```python
from build123d import *

# Parameters (mm, degrees)
SKETCH1_R           = 2.6
SKETCH1_R_2         = 7.6
BOSS_EXTRUDE1_DEPTH = 1.8
FILLET1_R           = 3
FILLET2_R           = 1.4
SCALE1_SCALE        = 1.15


with BuildPart() as part:
    # Sketch1 → Boss-Extrude1 (new body)
    with BuildSketch(Plane(origin=(0, 0, 0), x_dir=(1, 0, 0), z_dir=(0, 1, 0))):
        Polygon((20.3, 35.160631394), (-20.3, 35.160631394), (-40.6, 0), (-20.3, -35.160631394), (20.3, -35.160631394), (40.6, 0), align=None)
        with Locations((-18.636201283, -32.21652123)):
            Circle(SKETCH1_R, mode=Mode.SUBTRACT)
        with Locations((18.582225165, -32.247684356)):
            Circle(SKETCH1_R, mode=Mode.SUBTRACT)
        with Locations((37.218426448, -0.031163126)):
            Circle(SKETCH1_R, mode=Mode.SUBTRACT)
        with Locations((-37.218426448, 0.031163126)):
            Circle(SKETCH1_R, mode=Mode.SUBTRACT)
        with BuildLine():
            Line((-32.142053523, 3.218057696), (-18.857946477, 26.226806032))
            Line((-18.857946477, 26.226806032), (-10.521325069, 11.78735419))
            ThreePointArc((-10.521325069, 11.78735419), (-13.68320138, 7.9), (-15.468810706, 3.218057696))
            Line((-15.468810706, 3.218057696), (-32.142053523, 3.218057696))
        make_face(mode=Mode.SUBTRACT)
        with BuildLine():
            Line((-18.857946477, -26.226806032), (-32.142053523, -3.218057696))
            Line((-32.142053523, -3.218057696), (-15.468810706, -3.218057696))
            ThreePointArc((-15.468810706, -3.218057696), (-13.68320138, -7.9), (-10.521325069, -11.78735419))
            Line((-10.521325069, -11.78735419), (-18.857946477, -26.226806032))
        make_face(mode=Mode.SUBTRACT)
        with BuildLine():
            Line((13.284107046, -29.444863729), (-13.284107046, -29.444863729))
            Line((-13.284107046, -29.444863729), (-4.947485637, -15.005411886))
            ThreePointArc((-4.947485637, -15.005411886), (0, -15.8), (4.947485637, -15.005411886))
            Line((4.947485637, -15.005411886), (13.284107046, -29.444863729))
        make_face(mode=Mode.SUBTRACT)
        with BuildLine():
            Line((32.142053523, -3.218057696), (18.857946477, -26.226806032))
            Line((18.857946477, -26.226806032), (10.521325069, -11.78735419))
            ThreePointArc((10.521325069, -11.78735419), (13.68320138, -7.9), (15.468810706, -3.218057696))
            Line((15.468810706, -3.218057696), (32.142053523, -3.218057696))
        make_face(mode=Mode.SUBTRACT)
        with BuildLine():
            Line((18.857946477, 26.226806032), (32.142053523, 3.218057696))
            Line((32.142053523, 3.218057696), (15.468810706, 3.218057696))
            ThreePointArc((15.468810706, 3.218057696), (13.68320138, 7.9), (10.521325069, 11.78735419))
            Line((10.521325069, 11.78735419), (18.857946477, 26.226806032))
        make_face(mode=Mode.SUBTRACT)
        with BuildLine():
            Line((-13.284107046, 29.444863729), (13.284107046, 29.444863729))
            Line((13.284107046, 29.444863729), (4.947485637, 15.005411886))
            ThreePointArc((4.947485637, 15.005411886), (0, 15.8), (-4.947485637, 15.005411886))
            Line((-4.947485637, 15.005411886), (-13.284107046, 29.444863729))
        make_face(mode=Mode.SUBTRACT)
        with Locations((-18.582225165, 32.247684356)):
            Circle(SKETCH1_R, mode=Mode.SUBTRACT)
        with Locations((18.636201283, 32.21652123)):
            Circle(SKETCH1_R, mode=Mode.SUBTRACT)
        with Locations((0.052857117, 0)):
            Circle(SKETCH1_R_2, mode=Mode.SUBTRACT)
    extrude(amount=BOSS_EXTRUDE1_DEPTH)

    # Fillet1
    fillet1_edges = [part.edges().sort_by_distance(p)[0] for p in [
        (40.6, 0.9, 0),
        (20.3, 0.9, 35.160631394),
        (-20.3, 0.9, 35.160631394),
        (-40.6, 0.9, 0),
        (-20.3, 0.9, -35.160631394),
        (20.3, 0.9, -35.160631394),
    ]]
    fillet(fillet1_edges, radius=FILLET1_R)

    # Fillet2
    fillet2_edges = [part.edges().sort_by_distance(p)[0] for p in [
        (-32.142053523, 0.9, -3.218057696),
        (-15.468810706, 0.9, -3.218057696),
        (-10.521325069, 0.9, -11.78735419),
        (-18.857946477, 0.9, -26.226806032),
        (-18.857946477, 0.9, 26.226806032),
        (-10.521325069, 0.9, 11.78735419),
        (-15.468810706, 0.9, 3.218057696),
        (-32.142053523, 0.9, 3.218057696),
        (13.284107046, 0.9, 29.444863729),
        (4.947485637, 0.9, 15.005411886),
        (-4.947485637, 0.9, 15.005411886),
        (-13.284107046, 0.9, 29.444863729),
        (32.142053523, 0.9, 3.218057696),
        (15.468810706, 0.9, 3.218057696),
        (10.521325069, 0.9, 11.78735419),
        (18.857946477, 0.9, 26.226806032),
        (18.857946477, 0.9, -26.226806032),
        (10.521325069, 0.9, -11.78735419),
        (15.468810706, 0.9, -3.218057696),
        (32.142053523, 0.9, -3.218057696),
        (-13.284107046, 0.9, -29.444863729),
        (-4.947485637, 0.9, -15.005411886),
        (4.947485637, 0.9, -15.005411886),
        (13.284107046, 0.9, -29.444863729),
    ]]
    fillet(fillet2_edges, radius=FILLET2_R)


with BuildPart() as part_1:
    # Scale1: scaled about (-0.003928135, 0.9, 0)
    add(part.part.scale(SCALE1_SCALE).moved(Location((0.00058922, -0.135, 0))))


solid = part_1.part
```
Here's how the part is built. I have some questions about the finished solid (model axes, mm). A direction names the side the tool comes from. Coordinates: 2 decimals unless noted, no trailing zeros. Loops run counter-clockwise (first coordinate to the right, second up) from the corner with the lowest first, then second, coordinate; pieces in that order, holes last. Notation, with made-up numbers: M 11.25,-19.5 L 15.25,-19.5 A20 ccw 15.25,-7.5 Z; hole C -32,2.5 d9. An arc over 180 degrees is marked long. One line per item, written item: value.
1. Will these pins go through, and if not, where does the flat tip stop? pin 1 Ø0.6 at (x, y) = (-25, 1) entering from -Z; pin 2 Ø1 at (x, y) = (23.5, 1.5) entering from -Z; pin 3 Ø1 at (x, y) = (35.5, 0.5) entering from +Z.
Geometry says:
pin 1: stops at z = -38.09
pin 2: stops at z = -40.02
pin 3: stops at z = 20.25
2. Imagine slicing it at A-A (x = -11.5). List the corners of the cut face in (y, z) for me (3 decimals), and give its area (3 significant figures).
Geometry says:
outline: M -0.135,-40.435 L 1.935,-40.435 L 1.935,-33.862 L -0.135,-33.862 Z; M -0.135,-27.321 L 1.935,-27.321 L 1.935,27.321 L -0.135,27.321 Z; M -0.135,33.862 L 1.935,33.862 L 1.935,40.435 L -0.135,40.435 Z
area: 140 mm2
3. Imagine slicing it at B-B (z = -23). List the corners of the cut face in (x, y) for me (3 decimals), and give its area (3 significant figures).
Geometry says:
outline: M -33.41,-0.135 L -25.82,-0.135 L -25.82,1.935 L -33.41,1.935 Z; M -17.552,-0.135 L -9.005,-0.135 L -9.005,1.935 L -17.552,1.935 Z; M 9.006,-0.135 L 17.553,-0.135 L 17.553,1.935 L 9.006,1.935 Z; M 25.822,-0.135 L 33.412,-0.135 L 33.412,1.935 L 25.822,1.935 Z
area: 66.8 mm2
4. Imagine slicing it at C-C (x = 10). List the corners of the cut face in (y, z) for me (3 decimals), and give its area (3 significant figures).
Geometry says:
outline: M -0.135,-40.435 L 1.935,-40.435 L 1.935,-33.862 L -0.135,-33.862 Z; M -0.135,-24.721 L 1.935,-24.721 L 1.935,24.721 L -0.135,24.721 Z; M -0.135,33.862 L 1.935,33.862 L 1.935,40.435 L -0.135,40.435 Z
area: 130 mm2
5. Please list where these lines run through material, in increasing order: probe 1 along X at (y, z) = (1.4, 0); probe 2 along Z at (x, y) = (-29.5, 1.55); probe 3 along Z at (x, y) = (19, 0.45).
Geometry says:
probe 1: x = -46.16 to -45.79, -39.81 to -8.68, 8.8 to 39.81, 45.79 to 46.16
probe 2: z = -29.77 to -16.63, -3.7 to 3.7, 16.63 to 29.77
probe 3: z = -40.43 to -38.79, -35.31 to -25.51, -3.7 to 3.7, 25.51 to 35.26, 38.91 to 40.43
6. On a 3-axis mill with a long thin cutter (end or side, diameter ignored), from which of +Z, -Z, +X, -X, +Y, -Y can I reach the whole of each face in a straight line? I mean faces 4 (the cylindrical face through (15.77, 0.89, -9.03)), 5 (the cylindrical face through (46.157, 0.914, -0.025)). Say none if no direction works.
Geometry says:
face 4: +Y, -Y
face 5: +X, +Y, -Y
7. Thinking about a two-plate mould opening in X: for faces 1 (the flat face through (35.168, 0.886, -19.958)), 2 (the flat face through (27, 1, 3.701)), 3 (the cylindrical face through (-23.056, 0.914, -39.985)), which applies, +X half, -X half, draft (parallel to the pull), parting line (faces both ways), or undercut?
Geometry says:
face 1: +X half
face 2: undercut
face 3: -X half
8. Imagine slicing it at D-D (y = 1.45). State how many separate pieces and enclosed holes the cut face has, and give its area (3 significant figures).
Geometry says:
separate pieces: 1
enclosed holes: 13
area: 3,230 mm2
